from build123d import *

# Parameters (mm, degrees)
SKETCH1_R                = 4.1
BOSS_EXTRUDE1_DEPTH      = 3.5
BOSS_EXTRUDE2_DEPTH      = 51.7
BOSS_EXTRUDE2_DEPTH_BACK = 3.5
CHAMFER2_SIZE            = 5
CUT_EXTRUDE1_REACH       = 112.079
SKETCH4_W                = 51.7
SKETCH4_H                = 45
BOSS_EXTRUDE3_START      = 3.5
SKETCH5_R                = 4.1
BOSS_EXTRUDE3_DEPTH      = 3.5
CUT_EXTRUDE3_REACH       = 104.062
SKETCH9_R                = 1.35
SKETCH10_W               = 58.7
SKETCH10_H               = 53
BOSS_EXTRUDE5_DEPTH      = 3.175
SKETCH26_R               = 7.1
CUT_EXTRUDE6_DEPTH       = 4
SKETCH27_W               = 3.175
SKETCH27_H               = 34.600130378
BOSS_EXTRUDE6_DEPTH      = 45.22
SKETCH29_R               = 4.1
BOSS_EXTRUDE8_DEPTH      = 5.5
CHAMFER3_SIZE            = 3.175
BOSS_EXTRUDE9_START      = 10
SKETCH30_R               = 8
SKETCH30_R_2             = 4.1
BOSS_EXTRUDE9_DEPTH      = 10
SKETCH31_R               = 0.95
CUT_EXTRUDE7_DEPTH       = 120.972242206
BOSS_EXTRUDE10_DEPTH     = 45.22
SKETCH33_W               = 5.386290257
SKETCH33_H               = 2.7
BOSS_EXTRUDE11_DEPTH     = 45.22
BOSS_EXTRUDE12_DEPTH     = 0.2


with BuildPart() as part:
    # Sketch1 → Boss-Extrude1 (new body)
    with BuildSketch(Plane(origin=(0, 0, 0), x_dir=(0, 0, -1), z_dir=(1, 0, 0))):
        with BuildLine():
            Line((-17.5, 0), (-17.5, -20))
            Line((-17.5, -20), (-22.5, -20))
            Line((-22.5, -20), (-22.5, -76))
            Line((-22.5, -76), (22.5, -76))
            Line((22.5, -76), (22.5, -20))
            Line((22.5, -20), (17.5, -20))
            Line((17.5, -20), (17.5, 0))
            ThreePointArc((17.5, 0), (0, 17.5), (-17.5, 0))
        make_face()
        Circle(SKETCH1_R, mode=Mode.SUBTRACT)
    extrude(amount=-BOSS_EXTRUDE1_DEPTH)

    # Sketch2 → Boss-Extrude2 (add, two sides: drawn at the far end of the back side and taken through both)
    with BuildSketch(Plane(origin=(0, 0, 0), x_dir=(0, 0, -1), z_dir=(1, 0, 0)).offset(-BOSS_EXTRUDE2_DEPTH_BACK)):
        Polygon((-22.5, -20), (-22.5, -76), (22.5, -76), (22.5, -20), (26.5, -20), (26.5, -79.175), (-26.5, -79.175), (-26.5, -20), align=None)
    extrude(amount=BOSS_EXTRUDE2_DEPTH + BOSS_EXTRUDE2_DEPTH_BACK)

    # Chamfer2
    chamfer2_edges = [part.edges().sort_by_distance(p)[0] for p in [
        (24.1, -20, -26.5),
        (24.1, -20, 26.5),
    ]]
    chamfer(chamfer2_edges, length=CHAMFER2_SIZE)

    # Sketch4 → Cut-Extrude1 (cut, up to next)
    with BuildSketch(Plane(origin=(0, -76, 0), x_dir=(1, 0, 0), z_dir=(0, 1, 0)), mode=Mode.PRIVATE) as cut_extrude1_sk1:
        with Locations((25.85, 0)):
            Rectangle(SKETCH4_W, SKETCH4_H)
    cut_extrude1_tool1 = extrude(cut_extrude1_sk1.sketch, amount=-CUT_EXTRUDE1_REACH, mode=Mode.PRIVATE) & part.part
    add(cut_extrude1_tool1.solids().sort_by_distance((25.85, -76, 0))[0], mode=Mode.SUBTRACT)

    # Sketch5 → Boss-Extrude3 (add)
    with BuildSketch(Plane(origin=(51.7, 0, 0), x_dir=(0, 0, -1), z_dir=(1, 0, 0)).offset(BOSS_EXTRUDE3_START)):
        with BuildLine():
            Line((21.5, -20), (17.5, -20))
            Line((17.5, -20), (17.5, 0))
            ThreePointArc((17.5, 0), (0, 17.5), (-17.5, 0))
            Line((-17.5, 0), (-17.5, -20))
            Line((-17.5, -20), (-21.5, -20))
            Line((-21.5, -20), (-26.5, -25))
            Line((-26.5, -25), (-26.5, -79.175))
            Line((-26.5, -79.175), (26.5, -79.175))
            Line((26.5, -79.175), (26.5, -25))
            Line((26.5, -25), (21.5, -20))
        make_face()
        Circle(SKETCH5_R, mode=Mode.SUBTRACT)
    extrude(amount=-BOSS_EXTRUDE3_DEPTH)

    # Sketch9 → Cut-Extrude3 (cut, up to next)
    with BuildSketch(Plane(origin=(55.2, 0, 0), x_dir=(0, 0, -1), z_dir=(1, 0, 0)), mode=Mode.PRIVATE) as cut_extrude3_sk1:
        with Locations((0, 8.125)):
            Circle(SKETCH9_R)
    cut_extrude3_tool1 = extrude(cut_extrude3_sk1.sketch, amount=-CUT_EXTRUDE3_REACH, mode=Mode.PRIVATE) & part.part
    # Sketch9 → Cut-Extrude3 (cut, up to next)
    with BuildSketch(Plane(origin=(55.2, 0, 0), x_dir=(0, 0, -1), z_dir=(1, 0, 0)), mode=Mode.PRIVATE) as cut_extrude3_sk2:
        with Locations((8.125, 0)):
            Circle(SKETCH9_R)
    cut_extrude3_tool2 = extrude(cut_extrude3_sk2.sketch, amount=-CUT_EXTRUDE3_REACH, mode=Mode.PRIVATE) & part.part
    # Sketch9 → Cut-Extrude3 (cut, up to next)
    with BuildSketch(Plane(origin=(55.2, 0, 0), x_dir=(0, 0, -1), z_dir=(1, 0, 0)), mode=Mode.PRIVATE) as cut_extrude3_sk3:
        with Locations((0, -8.125)):
            Circle(SKETCH9_R)
    cut_extrude3_tool3 = extrude(cut_extrude3_sk3.sketch, amount=-CUT_EXTRUDE3_REACH, mode=Mode.PRIVATE) & part.part
    # Sketch9 → Cut-Extrude3 (cut, up to next)
    with BuildSketch(Plane(origin=(55.2, 0, 0), x_dir=(0, 0, -1), z_dir=(1, 0, 0)), mode=Mode.PRIVATE) as cut_extrude3_sk4:
        with Locations((-8.125, 0)):
            Circle(SKETCH9_R)
    cut_extrude3_tool4 = extrude(cut_extrude3_sk4.sketch, amount=-CUT_EXTRUDE3_REACH, mode=Mode.PRIVATE) & part.part
    add(cut_extrude3_tool1.solids().sort_by_distance((55.2, 8.125, 0))[0], mode=Mode.SUBTRACT)
    add(cut_extrude3_tool2.solids().sort_by_distance((55.2, 0, -8.125))[0], mode=Mode.SUBTRACT)
    add(cut_extrude3_tool3.solids().sort_by_distance((55.2, -8.125, 0))[0], mode=Mode.SUBTRACT)
    add(cut_extrude3_tool4.solids().sort_by_distance((55.2, 0, 8.125))[0], mode=Mode.SUBTRACT)

    # Sketch10 → Boss-Extrude5 (add)
    with BuildSketch(Plane.XZ.offset(79.175)):
        with Locations((25.85, 0)):
            Rectangle(SKETCH10_W, SKETCH10_H)
    extrude(amount=BOSS_EXTRUDE5_DEPTH)

    # Sketch26 → Cut-Extrude6 (cut)
    with BuildSketch(Plane.XY.offset(26.5)):
        with Locations((25.85, -69.065)):
            Circle(SKETCH26_R)
    extrude(amount=-CUT_EXTRUDE6_DEPTH, mode=Mode.SUBTRACT)

    # Sketch27 → Boss-Extrude6 (add)
    with BuildSketch(Plane(origin=(0, -79.175, 0), x_dir=(1, 0, 0), z_dir=(0, 1, 0))):
        with Locations((39.993724488, -5.199934811)):
            Rectangle(SKETCH27_W, SKETCH27_H)
        with Locations((11.706275512, -5.199934811)):
            Rectangle(SKETCH27_W, SKETCH27_H)
    extrude(amount=BOSS_EXTRUDE6_DEPTH)

    # Sketch29 → Boss-Extrude8 (add)
    with BuildSketch(Plane(origin=(0, 0, -26.5), x_dir=(-1, 0, 0), z_dir=(0, 0, -1))):
        with BuildLine():
            Line((-40.997321429, -82.35), (-55.2, -82.35))
            Line((-55.2, -82.35), (-31.95, -117.07))
            ThreePointArc((-31.95, -117.07), (-25.85, -123.17), (-19.75, -117.07))
            Line((-19.75, -117.07), (3.5, -82.35))
            Line((3.5, -82.35), (-10.702678571, -82.35))
            Line((-10.702678571, -82.35), (-10.702678571, -88.35))
            Line((-10.702678571, -88.35), (-20.85, -103.503333333))
            Line((-20.85, -103.503333333), (-30.85, -103.503333333))
            Line((-30.85, -103.503333333), (-40.997321429, -88.35))
            Line((-40.997321429, -88.35), (-40.997321429, -82.35))
        make_face()
        with Locations(Location((-25.85, -117.07, 0), (0, 0, 90))):
            Circle(SKETCH29_R, mode=Mode.SUBTRACT)
    extrude(amount=-BOSS_EXTRUDE8_DEPTH)

    # Chamfer3
    chamfer3_edges = [part.edges().sort_by_distance(p)[0] for p in [
        (43.575, -99.71, -26.5),
        (8.125, -99.71, -26.5),
        (-3.5, -53.675, -26.5),
        (-3.5, -53.675, 26.5),
        (55.2, -53.675, 26.5),
        (55.2, -53.675, -26.5),
    ]]
    chamfer(chamfer3_edges, length=CHAMFER3_SIZE)

    # Sketch30 → Boss-Extrude9 (add)
    with BuildSketch(Plane(origin=(0, 0, 0), x_dir=(0, 0, -1), z_dir=(1, 0, 0)).offset(BOSS_EXTRUDE9_START)):
        Circle(SKETCH30_R)
        Circle(SKETCH30_R_2, mode=Mode.SUBTRACT)
    extrude(amount=-BOSS_EXTRUDE9_DEPTH)

    # Sketch31 → Cut-Extrude7 (cut, through all)
    with BuildSketch(Plane(origin=(0, -20, 0), x_dir=(1, 0, 0), z_dir=(0, 1, 0))):
        with Locations(Location((5, 0, 0), (0, 0, 90))):
            Circle(SKETCH31_R)
    extrude(amount=CUT_EXTRUDE7_DEPTH, mode=Mode.SUBTRACT)

    # Sketch32 → Boss-Extrude10 (add)
    with BuildSketch(Plane(origin=(0, -79.175, 0), x_dir=(1, 0, 0), z_dir=(0, 1, 0))):
        Polygon((13.293775512, 12.600036526), (16.4, 12.600036526), (16.4, 15.600130378), (10.118775512, 15.600130378), (10.118775512, 12.100130378), (13.293775512, 12.100130378), align=None)
    boss_extrude10 = extrude(amount=BOSS_EXTRUDE10_DEPTH)

    # Sketch33 → Boss-Extrude11 (add)
    with BuildSketch(Plane(origin=(0, -79.175, 0), x_dir=(1, 0, 0), z_dir=(0, 1, 0))):
        with Locations((15.986920641, -21.15)):
            Rectangle(SKETCH33_W, SKETCH33_H)
    boss_extrude11 = extrude(amount=BOSS_EXTRUDE11_DEPTH)

    # Mirror1: Boss-Extrude10, Boss-Extrude11 across plane
    add(boss_extrude10.mirror(Plane.ZY.offset(-25.85)))
    add(boss_extrude11.mirror(Plane.ZY.offset(-25.85)))

    # Sketch34 → Boss-Extrude12 (add)
    with BuildSketch(Plane(origin=(0, -33.955, 0), x_dir=(1, 0, 0), z_dir=(0, 1, 0))):
        Polygon((13.293775512, -19.8), (13.293775512, 12.600036526), (16.4, 12.600036526), (16.4, 15.600130378), (10.118775512, 15.600130378), (10.118775512, -22.5), (18.680065769, -22.5), (18.680065769, -19.8), align=None)
        Polygon((41.581224488, -22.5), (41.581224488, 15.600130378), (35.3, 15.600130378), (35.3, 12.600036526), (38.406224488, 12.600036526), (38.406224488, -19.8), (33.019934231, -19.8), (33.019934231, -22.5), align=None)
    extrude(amount=BOSS_EXTRUDE12_DEPTH)


with BuildPart() as body_2:
    # Mirror3: mirrored copy
    add(part.part.mirror(Plane.ZY.offset(13.5)))


solid = body_2.part
Geometry check sheet. Reference: the model listing, model coordinates, mm. A direction names the side the tool comes from. Give positions to 0.01 mm unless a question says otherwise; leave off trailing zeros. Order: outer loops, then holes, each group sorted by start corner. A loop starts at its lowest first (then second) coordinate and runs counter-clockwise, first axis right, second up. Notation, with made-up numbers: (38.25, 83) - (55.25, 83) arc R14 ccw to (55.25, 104) - close; hole circle Ø8 at (-26, 4). An arc over 180 degrees is marked (long way). Answer as a JSON object with one key per item and string values.
(1) Cross-section at B-B (y = -28). Record the cut outline in (x, z) (3 decimals).
Report:
{"outline": "(-82.2, -23.325) - (-79.025, -26.5) - (-26.675, -26.5) - (-23.5, -23.325) - (-23.5, 23.325) - (-26.675, 26.5) - (-79.025, 26.5) - (-82.2, 23.325) - close; hole (-78.7, -22.5) - (-27, -22.5) - (-27, 22.5) - (-78.7, 22.5) - close"}
(2) Tool access check on faces 1 (the flat face through (-42.705, -95.821, -23.788)), 2 (the flat face through (-52, -50, -22.5)), 3 (the flat face through (-37, 2, 4)), 4 (the flat face through (-80, -20, -20)). Record the directions out of +Z, -Z, +X, -X, +Y, -Y that give a thin tool (end or side, any length) a straight path to the whole face; none if there is none.
Report:
{"face 1": "+Z, -Z", "face 2": "+Y", "face 3": "+Z, -Z, +Y", "face 4": "-Z, +X, -X, +Y"}
(3) Cross-section at A-A (x = -52.85). Record the cut outline in (y, z) (3 decimals).
Report:
{"outline": "(-123.17, -26.5) - (-121.17, -26.5) - (-121.17, -21) - (-123.17, -21) - close; (-112.97, -26.5) - (-103.503, -26.5) - (-103.503, -21) - (-112.97, -21) - close; (-82.35, -26.5) - (-25, -26.5) - (-21, -22.5) - (-79.175, -22.5) - (-79.175, 22.5) - (-76.165, 22.5) - (-76.165, 26.5) - (-82.35, 26.5) - close; (-61.965, 22.5) - (-21, 22.5) - (-25, 26.5) - (-61.965, 26.5) - close"}
(4) Cross-section at C-C (y = -60.5). Record the cut outline in (x, z) (3 decimals).
Report:
{"outline": "(-82.2, -23.325) - (-79.025, -26.5) - (-26.675, -26.5) - (-23.5, -23.325) - (-23.5, 23.325) - (-26.675, 26.5) - (-79.025, 26.5) - (-82.2, 23.325) - close; hole (-78.7, -22.5) - (-27, -22.5) - (-27, 22.5) - (-37.119, 22.5) - (-37.119, -15.6) - (-43.4, -15.6) - (-43.4, -12.6) - (-40.294, -12.6) - (-40.294, 19.8) - (-45.68, 19.8) - (-45.68, 22.5) - (-60.02, 22.5) - (-60.02, 19.8) - (-65.406, 19.8) - (-65.406, -12.6) - (-62.3, -12.6) - (-62.3, -15.6) - (-68.581, -15.6) - (-68.581, 22.5) - (-78.7, 22.5) - close"}
(5) Cross-section at D-D (z = 16). Record the cut outline in (x, y) (3 decimals), then the cut area to 3 significant figures.
Report:
{"outline": "(-82.2, -82.35) - (-23.5, -82.35) - (-23.5, 7.089) - (-27, 7.089) - (-27, -79.175) - (-37.119, -79.175) - (-37.119, -33.755) - (-40.294, -33.755) - (-40.294, -79.175) - (-65.406, -79.175) - (-65.406, -33.755) - (-68.581, -33.755) - (-68.581, -79.175) - (-78.7, -79.175) - (-78.7, 7.089) - (-82.2, 7.089) - close", "area": "1,080 mm^2"}
(6) Draft check along Z on faces 5 (the flat face through (-66, -33.755, 3)), 6 (the flat face through (-80.635, -52.511, 24.89)), 7 (the flat face through (-80.635, -51.664, -24.89)). Enter one of: released by +Z, released by -Z, zero draft, split by the parting line, or undercut.
Report:
{"face 5": "undercut", "face 6": "released by +Z", "face 7": "released by -Z"}
(7) Material ranges on line 1 (X direction, y = 6, z = 0); line 2 (X direction, y = -69, z = -12.5); line 3 (X direction, y = 6, z = -2.5), recorded low to high.
Report:
{"line 1": "-82.2 to -78.7, -37 to -32.95, -31.05 to -23.5", "line 2": "-82.2 to -78.7, -68.58 to -65.41, -40.29 to -37.12, -27 to -23.5", "line 3": "-82.2 to -78.7, -37 to -23.5"}
(8) Depth check by flat-ended pin: pin 1 Ø5 at (y, z) = (0, 0) entering from -X; pin 2 Ø9.5 at (x, z) = (-41, 7.5) entering from +Y; pin 3 Ø6 at (x, z) = (-54.5, -2.5) entering from +Y (3 decimals); pin 4 Ø6 at (y, z) = (-85, -24.5) entering from +X. Enter the tip coordinate at first touch or a pass-through.
Report:
{"pin 1": "through", "pin 2": "y = 6.29", "pin 3": "y = -79.175", "pin 4": "x = -23.5"}
